from build123d import *

# Parameters (mm, degrees)
SKICA1_W                = 245
SKICA1_H                = 85
SKICA1_W_2              = 102.5
SKICA1_H_2              = 27
SKICA1_W_3              = 71
SKICA1_H_3              = 10.5
P_IDAT_VYSUNUT_M1_DEPTH = 3
SKICA2_W                = 3
SKICA2_H                = 25
SKICA2_W_2              = 25
SKICA2_H_2              = 3
P_IDAT_VYSUNUT_M2_DEPTH = 3
SKICA3_W                = 5
SKICA3_H                = 3
P_IDAT_VYSUNUT_M3_DEPTH = 3
ZAOBLIT1_R              = 5
SKICA7_W                = 5
SKICA7_H                = 3
P_IDAT_VYSUNUT_M6_DEPTH = 3


with BuildPart() as part:
    # Skica1 → Přidat vysunutím1 (new body)
    with BuildSketch(Plane(origin=(0, 0, 0), x_dir=(1, 0, 0), z_dir=(0, 1, 0))):
        with Locations((122.5, 42.5)):
            Rectangle(SKICA1_W, SKICA1_H)
        with Locations((71.25, 23.833333333)):
            Rectangle(SKICA1_W_2, SKICA1_H_2, mode=Mode.SUBTRACT)
        with Locations((55.5, 69.416666667)):
            Rectangle(SKICA1_W_3, SKICA1_H_3, mode=Mode.SUBTRACT)
        with Locations((183.75, 23.833333333)):
            Rectangle(SKICA1_W_2, SKICA1_H_2, mode=Mode.SUBTRACT)
        with Locations((183.75, 61.166666667)):
            Rectangle(SKICA1_W_2, SKICA1_H_2, mode=Mode.SUBTRACT)
        with BuildLine():
            Line((102.5, 74.666666667), (115.5, 74.666666667))
            ThreePointArc((115.5, 74.666666667), (120.449747468, 72.616414135), (122.5, 67.666666667))
            Line((122.5, 67.666666667), (122.5, 54.666666667))
            ThreePointArc((122.5, 54.666666667), (120.449747468, 49.716919198), (115.5, 47.666666667))
            Line((115.5, 47.666666667), (102.5, 47.666666667))
            ThreePointArc((102.5, 47.666666667), (97.550252532, 49.716919198), (95.5, 54.666666667))
            Line((95.5, 54.666666667), (95.5, 67.666666667))
            ThreePointArc((95.5, 67.666666667), (97.550252532, 72.616414135), (102.5, 74.666666667))
        make_face(mode=Mode.SUBTRACT)
        with Locations((55.5, 52.916666667)):
            Rectangle(SKICA1_W_3, SKICA1_H_3, mode=Mode.SUBTRACT)
    extrude(amount=P_IDAT_VYSUNUT_M1_DEPTH)

    # Skica2 → Přidat vysunutím2 (add)
    with BuildSketch(Plane(origin=(0, 0, 0), x_dir=(1, 0, 0), z_dir=(0, 1, 0))):
        with Locations((-1.5, 17.5)):
            Rectangle(SKICA2_W, SKICA2_H)
        with Locations((-1.5, 67.5)):
            Rectangle(SKICA2_W, SKICA2_H)
        with Locations((232.5, -1.5)):
            Rectangle(SKICA2_W_2, SKICA2_H_2)
        with Locations((182.5, -1.5)):
            Rectangle(SKICA2_W_2, SKICA2_H_2)
        with Locations((132.5, -1.5)):
            Rectangle(SKICA2_W_2, SKICA2_H_2)
        with Locations((82.5, -1.5)):
            Rectangle(SKICA2_W_2, SKICA2_H_2)
        with Locations((32.5, -1.5)):
            Rectangle(SKICA2_W_2, SKICA2_H_2)
    extrude(amount=P_IDAT_VYSUNUT_M2_DEPTH)

    # Skica3 → Přidat vysunutím3 (add)
    with BuildSketch(Plane(origin=(0, 0, 0), x_dir=(1, 0, 0), z_dir=(0, 1, 0))):
        with Locations((7.5, 86.5)):
            Rectangle(SKICA3_W, SKICA3_H)
        with Locations((17.5, 86.5)):
            Rectangle(SKICA3_W, SKICA3_H)
    extrude(amount=P_IDAT_VYSUNUT_M3_DEPTH)

    # Zaoblit1
    zaoblit1_edges = [part.edges().sort_by_distance(p)[0] for p in [
        (245, 1.5, -85),
    ]]
    fillet(zaoblit1_edges, radius=ZAOBLIT1_R)

    # Skica7 → Přidat vysunutím6 (add)
    with BuildSketch(Plane(origin=(0, 0, 0), x_dir=(1, 0, 0), z_dir=(0, 1, 0))):
        with Locations((162.5, 86.5)):
            Rectangle(SKICA7_W, SKICA7_H)
        with Locations((172.5, 86.5)):
            Rectangle(SKICA7_W, SKICA7_H)
    extrude(amount=P_IDAT_VYSUNUT_M6_DEPTH)


solid = part.part
The listing builds one solid part. Answer for the finished solid, in the listing's coordinates (mm). A direction names the side the tool comes from. Round coordinates to 2 decimals unless told otherwise and drop trailing zeros. Loops run counter-clockwise (first coordinate to the right, second up) from the corner with the lowest first, then second, coordinate; pieces in that order, holes last. Notation, with made-up numbers: M 77,35.25 L 116,35.25 A21 cw 116,72.25 Z; hole C 25.5,-21.5 d6. An arc over 180 degrees is marked long. Return JSON: item names as keys, results as strings.
Q1. Find section B-B, the plane y = 1.9. State how many separate pieces and enclosed holes the cut face has, plus the area to 3 significant figures.
Results list:
{"separate pieces": "1", "enclosed holes": "6", "area": "10,900 mm2"}
Q2. The mould has two halves that part along X. Classify faces 3 (the face through (97.496, 1.479, -72.562)), 4 (the face through (92, 3, -43)), 5 (the face through (244, 2, -83)): released by +X, released by -X, zero draft, split by the parting line, or undercut.
Results list:
{"face 3": "undercut", "face 4": "zero draft", "face 5": "released by +X"}
Q3. Find section D-D, the plane x = 12.5. Determine the outline of the cut face in (y, z).
Results list:
{"outline": "M 0,-85 L 3,-85 L 3,0 L 0,0 Z"}
Q4. Each of these flat-tipped pins is pushed along its axis until it touches: pin 1 Ø1.5 at (x, y) = (208.5, 2) entering from +Z; pin 2 Ø1.5 at (x, y) = (41, 2) entering from -Z. Where does it stop, or does it pass through?
Results list:
{"pin 1": "stops at z = 0", "pin 2": "stops at z = -85"}
Q5. Find the intervals of material crossed by line 1 along X through (y, z) = (2.45, -68); line 2 along Z through (x, y) = (174.5, 2.7); line 3 along X through (y, z) = (2, -20), in increasing order. Write a range as from..to.
Results list:
{"line 1": "x = -3..20, 91..95.51, 122.49..132.5, 235..245", "line 2": "z = -88..-74.67, -47.67..-37.33, -10.33..3", "line 3": "x = -3..20, 122.5..132.5, 235..245"}
Q6. Find section C-C, the plane x = 182. Determine the outline of the cut face in (y, z), plus the area to 3 significant figures.
Results list:
{"outline": "M 0,-85 L 3,-85 L 3,-74.67 L 0,-74.67 Z; M 0,-47.67 L 3,-47.67 L 3,-37.33 L 0,-37.33 Z; M 0,-10.33 L 3,-10.33 L 3,3 L 0,3 Z", "area": "102 mm2"}
Q7. Which of the six approach directions +Z, -Z, +X, -X, +Y, -Y give full straight-line access (tool end or side, diameter ignored) to faces 1 (the face through (97.605, 1.479, -49.663)), 2 (the face through (92, 0, -43))?
Results list:
{"face 1": "+Y, -Y", "face 2": "+Z, -Z, +X, -X, -Y"}
Q8. Find section A-A, the plane x = 150. Determine the outline of the cut face in (y, z).
Results list:
{"outline": "M 0,-85 L 3,-85 L 3,-74.67 L 0,-74.67 Z; M 0,-47.67 L 3,-47.67 L 3,-37.33 L 0,-37.33 Z; M 0,-10.33 L 3,-10.33 L 3,0 L 0,0 Z"}
